Check sheet for the modelled part. Datum: model origin and axes. Units: mm. A direction names the side the tool comes from. Give positions to 0.01 mm unless a question says otherwise; leave off trailing zeros. Order: outer loops, then holes, each group sorted by start corner. A loop starts at its lowest first (then second) coordinate and runs counter-clockwise, first axis right, second up. Notation, with made-up numbers: M 28,75.25 L 73,75.25 A8 cw 73,82.25 Z; hole C 21,15.5 d7. An arc over 180 degrees is marked long. Answer in a Markdown table with one row per item. Add a question column.
from build123d import *

# Parameters (mm, degrees)
SKETCH1_R           = 1.6
SKETCH1_R_2         = 8
BOSS_EXTRUDE1_DEPTH = 5
FILLET1_R           = 10
FILLET2_R           = 10


with BuildPart() as part:
    # Sketch1 → Boss-Extrude1 (new body)
    with BuildSketch(Plane.XY):
        with BuildLine():
            Line((13, 9.327379053), (53, 9.327379053))
            Line((53, 9.327379053), (53, -9.327379053))
            Line((53, -9.327379053), (13, -9.327379053))
            ThreePointArc((13, -9.327379053), (-16, 0), (13, 9.327379053))
        make_face()
        with Locations((0, 13)):
            Circle(SKETCH1_R, mode=Mode.SUBTRACT)
        with Locations((9.192388155, 9.192388155)):
            Circle(SKETCH1_R, mode=Mode.SUBTRACT)
        with Locations((13, 0)):
            Circle(SKETCH1_R, mode=Mode.SUBTRACT)
        with Locations((9.192388155, -9.192388155)):
            Circle(SKETCH1_R, mode=Mode.SUBTRACT)
        with Locations((0, -13)):
            Circle(SKETCH1_R, mode=Mode.SUBTRACT)
        with Locations((-9.192388155, -9.192388155)):
            Circle(SKETCH1_R, mode=Mode.SUBTRACT)
        with Locations((-13, 0)):
            Circle(SKETCH1_R, mode=Mode.SUBTRACT)
        with Locations((-9.192388155, 9.192388155)):
            Circle(SKETCH1_R, mode=Mode.SUBTRACT)
        Circle(SKETCH1_R_2, mode=Mode.SUBTRACT)
    extrude(amount=BOSS_EXTRUDE1_DEPTH)

    # Fillet1
    # the kernel refuses this fillet: 10 mm, written as the material it takes off along each edge
    with BuildSketch(Plane(origin=(53, -9.327379053, -25), x_dir=(0, 1, 0), z_dir=(0, 0, 1)), Plane(origin=(53, 9.327379053, -25), x_dir=(-1, 0, 0), z_dir=(0, 0, 1))) as fillet1_piece_1:
        with BuildLine():
            CenterArc((FILLET1_R, FILLET1_R), FILLET1_R, 180, 90)
            Line((0, FILLET1_R), (0, 0))
            Line((0, 0), (FILLET1_R, 0))
        make_face()
    extrude(amount=55, mode=Mode.SUBTRACT)

    # Fillet2
    fillet2_edges = [part.edges().sort_by_distance(p)[0] for p in [
        (13, 9.327379053, 2.5),
        (13, -9.327379053, 2.5),
    ]]
    fillet(fillet2_edges, radius=FILLET2_R)


solid = part.part
Q1. Cross-section at A-A (x = -13). Record the boundary of the cut face in (y, z).
Q2. Draft check along X on faces 1 (the flat face through (19, 0, 5)), 2 (the cylindrical face through (-9.539, -10.754, 2.465)), 3 (the cylindrical face through (13.86, 9.97, 2.54)). Enter one of: pulls with the +X half, pulls with the -X half, needs draft (parallel to the pull), parting line crosses it, or undercut.
Q3. Tool access check on faces 4 (the flat face through (30, 9.327, 2)), 5 (the cylindrical face through (8.846, -10.754, 2.465)), 6 (the flat face through (30, -9.327, 2)). Record the directions out of +Z, -Z, +X, -X, +Y, -Y that give a thin tool (end or side, any length) a straight path to the whole face; none if there is none.
Q4. Thickness scan on probe 1 along Y at (x, z) = (0, 3.9); probe 2 along Y at (x, z) = (-13, 2.45); probe 3 along X at (y, z) = (-8.5, 0.3). Record the ranges inside material, lowest first.
Q5. Cross-section at C-C (x = 0). Record the boundary of the cut face in (y, z).
Q6. Cross-section at B-B (y = -5.5). Record the boundary of the cut face in (x, z).
Q7. Cross-section at D-D (z = 3.05). State how many separate pieces and enclosed holes the cut face has, and give its area (3 significant figures).
Q8. Go/stop test with flat-tipped pins: pin 1 (5 mm diameter, centred on x = 9.19, y = -9.19, fed in from -Z); pin 2 (1.5 mm diameter, centred on x = 33.5, z = 2, fed in from -Y); pin 3 (2 mm diameter, centred on x = -2.5, z = 1, fed in from +Y); pin 4 (2 mm diameter, centred on y = 8, z = 3.5, fed in from +X). Record where each tip stops, or that it passes through.
Values follow:
| question | item | result |
|---|---|---|
| 1 | outline | M -9.33,0 L -1.6,0 L -1.6,5 L -9.33,5 Z; M 1.6,0 L 9.33,0 L 9.33,5 L 1.6,5 Z |
| 2 | face 1 | needs draft |
| 2 | face 2 | undercut |
| 2 | face 3 | pulls with the +X half |
| 3 | face 4 | +Z, -Z, +X, +Y |
| 3 | face 5 | +Z, -Z |
| 3 | face 6 | +Z, -Z, +X, -Y |
| 4 | probe 1 | -16 to -14.6, -11.4 to -8, 8 to 11.4, 14.6 to 16 |
| 4 | probe 2 | -9.33 to -1.6, 1.6 to 9.33 |
| 4 | probe 3 | -13.56 to -10.63, -7.75 to 7.75, 10.63 to 46.98 |
| 5 | outline | M -16,0 L -14.6,0 L -14.6,5 L -16,5 Z; M -11.4,0 L -8,0 L -8,5 L -11.4,5 Z; M 8,0 L 11.4,0 L 11.4,5 L 8,5 Z; M 14.6,0 L 16,0 L 16,5 L 14.6,5 Z |
| 6 | outline | M -15.02,0 L -5.81,0 L -5.81,5 L -15.02,5 Z; M 5.81,0 L 50.87,0 L 50.87,5 L 5.81,5 Z |
| 7 | separate pieces | 1 |
| 7 | enclosed holes | 9 |
| 7 | area | 1,210 mm² |
| 8 | pin 1 | z = 0 |
| 8 | pin 2 | y = -9.33 |
| 8 | pin 3 | y = 15.93 |
| 8 | pin 4 | x = 49.41 |
